```python
from build123d import *

# Parameters (mm, degrees)
BOSS_EXTRUDE1_DEPTH = 6
FILLET1_R           = 4
FILLET2_R           = 2
SKETCH2_R           = 1.5
CUT_EXTRUDE1_DEPTH  = 6
CHAMFER1_SIZE       = 0.5


with BuildPart() as part:
    # Sketch1 → Boss-Extrude1 (new body)
    with BuildSketch(Plane(origin=(0, 0, 0), x_dir=(1, 0, 0), z_dir=(0, 1, 0))):
        Polygon((-10.4, 10.7), (-14.4, 2.7), (-14.4, -10.7), (14.4, -10.7), (14.4, 2.7), (10.4, 10.7), align=None)
    extrude(amount=BOSS_EXTRUDE1_DEPTH)

    # Fillet1
    fillet1_edges = [part.edges().sort_by_distance(p)[0] for p in [
        (14.4, 3, -2.7),
        (-14.4, 3, -2.7),
        (-10.4, 3, -10.7),
        (10.4, 3, -10.7),
    ]]
    fillet(fillet1_edges, radius=FILLET1_R)

    # Fillet2
    fillet2_edges = [part.edges().sort_by_distance(p)[0] for p in [
        (14.4, 3, 10.7),
        (-14.4, 3, 10.7),
    ]]
    fillet(fillet2_edges, radius=FILLET2_R)

    # Sketch2 → Cut-Extrude1 (cut)
    with BuildSketch(Plane.XZ):
        with Locations(Location((-8, 0, 0), (0, 0, 270))):
            Circle(SKETCH2_R)
        with Locations(Location((8, 0, 0), (0, 0, 270))):
            Circle(SKETCH2_R)
    extrude(amount=-CUT_EXTRUDE1_DEPTH, mode=Mode.SUBTRACT)

    # Chamfer1
    chamfer1_edges = [part.edges().sort_by_distance(p)[0] for p in [
        (12.741640786, 0, -6.016718427),
        (-12.741640786, 0, -6.016718427),
        (0, 0, -10.7),
        (10.030788493, 0, -10.102603233),
        (-10.030788493, 0, -10.102603233),
        (14.292995958, 0, -2.674739772),
        (-14.292995958, 0, -2.674739772),
        (-12.741640786, 6, -6.016718427),
        (12.741640786, 6, -6.016718427),
        (0, 6, -10.7),
        (10.030788493, 6, -10.102603233),
        (-10.030788493, 6, -10.102603233),
        (14.292995958, 6, -2.674739772),
        (-14.292995958, 6, -2.674739772),
        (14.4, 0, 3.472135955),
        (14.4, 6, 3.472135955),
        (-14.4, 0, 3.472135955),
        (0, 0, 10.7),
        (-13.814213562, 0, 10.114213562),
        (13.814213562, 0, 10.114213562),
        (0, 6, 10.7),
        (-14.4, 6, 3.472135955),
        (-13.814213562, 6, 10.114213562),
        (13.814213562, 6, 10.114213562),
    ]]
    chamfer(chamfer1_edges, length=CHAMFER1_SIZE)


solid = part.part
```
Could you check a few things on this model? Use its own coordinates, in mm. Give positions to 0.01 mm unless a question says otherwise; leave off trailing zeros. Loops run counter-clockwise (first coordinate to the right, second up) from the corner with the lowest first, then second, coordinate; pieces in that order, holes last. Notation, with made-up numbers: (50.25, 51) - (89.25, 51) arc R7 ccw to (89.25, 59) - close; hole circle Ø5 at (82.5, 70.25). An arc over 180 degrees is marked (long way). Answer in a Markdown table with one row per item. Add a question column.
Q1. If we section it at B-B (y = 3.5): List the corners of the cut face in (x, z) for me, plus the area to 3 significant figures.
Q2. If we section it at A-A (z = 0): List the corners of the cut face in (x, y) for me, plus the area to 3 significant figures.
Q3. Please list where these lines run through material, in increasing order: L1, parallel to X at y = 4.6, z = 0; L2, parallel to X at y = 3.75, z = 1; L3, parallel to Z at x = 8.25, y = 1. Write a range as from..to.
The answers:
| question | item | result |
|---|---|---|
| 1 | outline | (-14.4, -1.76) arc R4 ccw to (-13.98, -3.54) - (-11.51, -8.49) arc R4 ccw to (-7.93, -10.7) - (7.93, -10.7) arc R4 ccw to (11.51, -8.49) - (13.98, -3.54) arc R4 ccw to (14.4, -1.76) - (14.4, 8.7) arc R2 ccw to (12.4, 10.7) - (-12.4, 10.7) arc R2 ccw to (-14.4, 8.7) - close; hole circle Ø3 at (-8, 0); hole circle Ø3 at (8, 0) |
| 1 | area | 566 mm^2 |
| 2 | outline | (-14.4, 0.5) - (-13.9, 0) - (-9.5, 0) - (-9.5, 6) - (-13.9, 6) - (-14.4, 5.5) - close; (-6.5, 0) - (6.5, 0) - (6.5, 6) - (-6.5, 6) - close; (9.5, 0) - (13.9, 0) - (14.4, 0.5) - (14.4, 5.5) - (13.9, 6) - (9.5, 6) - close |
| 2 | area | 136 mm^2 |
| 3 | L1 | x = -14.4..-9.5, -6.5..6.5, 9.5..14.4 |
| 3 | L2 | x = -14.4..-9.12, -6.88..6.88, 9.12..14.4 |
| 3 | L3 | z = -10.69..-1.48, 1.48..10.7 |
